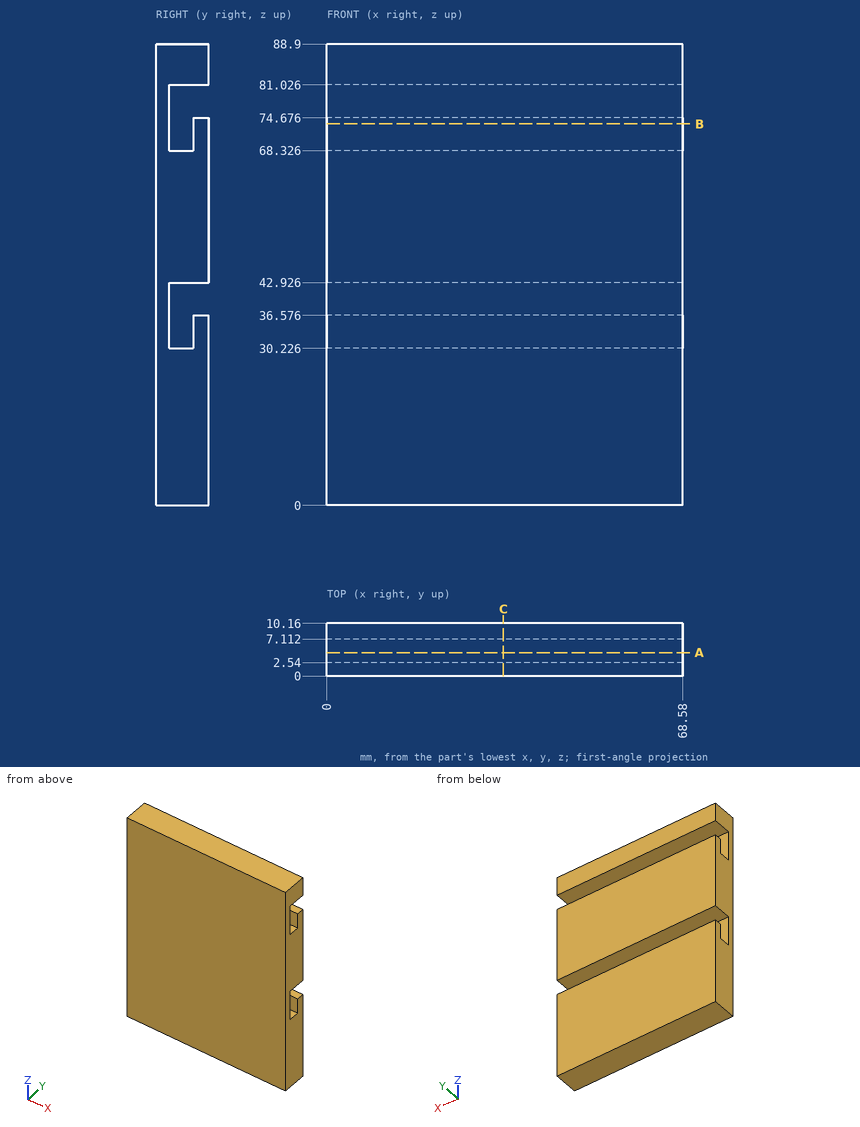
Source: three-view drawing plus pictorial views. Frame: mm from the lowest corner of the part. Round coordinates to 2 decimals unless told otherwise and drop trailing zeros. Loops run counter-clockwise (first coordinate to the right, second up) from the corner with the lowest first, then second, coordinate; pieces in that order, holes last.
Q1. First-contact query: P1, Ø14, axis at x = 27, z = 77.5, coming from the +Y side. Flat tip, straight axial feed; report the tip coordinate or a pass-through.
Q2. Section C-C, the plane x = 34. Return loops of the section in (y, z), plus the area to 3 significant figures.
Q3. Section B-B, the plane z = 73.5. Return loops of the section in (x, y), plus the area to 3 significant figures.
Q4. Ray query, line 1 (Z direction, x = 46, y = 3.5); line 2 (Z direction, x = 50, y = 7.75); line 3 (Y direction, x = 34.5, z = 75.5). Return the intervals inside material, ascending.
Q5. Section A-A, the plane y = 4.5. Return loops of the section in (x, z), plus the area to 3 significant figures.
Solutions:
1. P1: stops at y = 10.16
2. outline: (0, 0) - (10.16, 0) - (10.16, 36.58) - (7.11, 36.58) - (7.11, 30.23) - (2.54, 30.23) - (2.54, 42.93) - (10.16, 42.93) - (10.16, 74.68) - (7.11, 74.68) - (7.11, 68.33) - (2.54, 68.33) - (2.54, 81.03) - (10.16, 81.03) - (10.16, 88.9) - (0, 88.9) - close
2. area: 748 mm2
3. outline: (0, 0) - (68.58, 0) - (68.58, 2.54) - (0, 2.54) - close; (0, 7.11) - (68.58, 7.11) - (68.58, 10.16) - (0, 10.16) - close
3. area: 383 mm2
4. line 1: z = 0 to 30.23, 42.93 to 68.33, 81.03 to 88.9
4. line 2: z = 0 to 36.58, 42.93 to 74.68, 81.03 to 88.9
4. line 3: y = 0 to 2.54
5. outline: (0, 0) - (68.58, 0) - (68.58, 30.23) - (0, 30.23) - close; (0, 42.93) - (68.58, 42.93) - (68.58, 68.33) - (0, 68.33) - close; (0, 81.03) - (68.58, 81.03) - (68.58, 88.9) - (0, 88.9) - close
5. area: 4,350 mm2
